Autodesk Inventor part; units mm, degrees
ref_plane "YZ Plane" through (0, 0, 0) normal (1, 0, 0) x (0, 1, 0)
ref_plane "XZ Plane" through (0, 0, 0) normal (0, 1, 0) x (-1, 0, 0)
ref_plane "XY Plane" through (0, 0, 0) normal (0, 0, 1) x (1, 0, 0)
sketch "Sketch1" plane through (0, 0, 0) normal (0, 1, 0) x (-1, 0, 0)
  circle A0 centre (0, 0) radius 1.8
  circle A1 centre (0, 0) radius 2.5
  dimension "d1" = 3.6
  dimension "d7" = 5
extrude "Extrusion1" add sketch "Sketch1" along normal blind 4 contours A0 | A1
extrude "Extrusion2" cut sketch "Sketch1" along normal blind 1 contours A0
fillet "Fillet1" radius 0.5 1 edges at (2.5, 4, 0)
properties part number "button"
Here's how the part is built. I have some questions about the finished solid (model axes, mm). A direction names the side the tool comes from. Give positions to 0.01 mm unless a question says otherwise; leave off trailing zeros. Loops run counter-clockwise (first coordinate to the right, second up) from the corner with the lowest first, then second, coordinate; pieces in that order, holes last. Notation, with made-up numbers: M 53,14 L 64,14 A11 cw 64,28 Z; hole C 42,77.25 d1. An arc over 180 degrees is marked long. Use one line per item in the form item = value. Start each with the question number.
Q1. Which directions (+Z, -Z, +X, -X, +Y, -Y) give clear straight access to the entire face, cutting with the end or side of a thin tool? Please do faces 4 (the cylindrical face through (-1.717, 0.493, -0.541)), 5 (the flat face through (0, 4, 0)).
Q2. Thinking about a two-plate mould opening in X: for faces 1 (the flat face through (1, 0, 2)), 2 (the cylindrical face through (0.54, 1.73, 2.44)), 3 (the flat face through (0, 1, 0)), which applies, +X half, -X half, draft (parallel to the pull), parting line (faces both ways), or undercut?
Q3. Will these pins go through, and if not, where does the flat tip stop? pin 1 Ø2 at (y, z) = (3.5, 0.5) entering from +X; pin 2 Ø1.5 at (x, y) = (1.5, 1) entering from -Z; pin 3 Ø1.8 at (x, z) = (0, 0) entering from -Y.
Q4. If we section it at C-C (y = 1.65): Write out the boundary of the cut face in (x, z).
Q5. If we section it at A-A (x = 0): Write out the boundary of the cut face in (y, z), then the cut area to 3 significant figures.
Q6. If we section it at B-B (z = 0): Write out the boundary of the cut face in (x, y).
Q7. I need wall thicknesses on line 1 along Y through (x, z) = (1.15, -0.35); line 2 along X through (y, z) = (0.6, -0.7); line 3 along Z through (x, y) = (-1.65, 2.1). Which ranges of each line are inside material? Lowest first, please.
Taken from the geometry:
q1.face_4 = -Y
q1.face_5 = +Z, -Z, +X, -X, +Y
q2.face_1 = draft
q2.face_2 = parting line
q2.face_3 = undercut
q3.pin_1 = 2.5
q3.pin_2 = -2.38
q3.pin_3 = 1
q4.outline = C 0,0 d5
q5.outline = M 0,-2.5 L 3.5,-2.5 A0.5 ccw 4,-2 L 4,2 A0.5 ccw 3.5,2.5 L 0,2.5 L 0,1.8 L 1,1.8 L 1,-1.8 L 0,-1.8 Z
q5.area = 16.3 mm^2
q6.outline = M -2.5,0 L -1.8,0 L -1.8,1 L 1.8,1 L 1.8,0 L 2.5,0 L 2.5,3.5 A0.5 ccw 2,4 L -2,4 A0.5 ccw -2.5,3.5 Z
q7.line_1 = 1 to 4
q7.line_2 = -2.4 to -1.66, 1.66 to 2.4
q7.line_3 = -1.88 to 1.88
